Work out the finished part from the listing and answer in its coordinate system (mm). A direction names the side the tool comes from. Coordinates: 2 decimals unless noted, no trailing zeros. Loops run counter-clockwise (first coordinate to the right, second up) from the corner with the lowest first, then second, coordinate; pieces in that order, holes last. Notation, with made-up numbers: (13.5, -5.5) - (58.5, -5.5) arc R25 ccw to (58.5, 29.5) - close; hole circle Ø2 at (59.5, 47.5). An arc over 180 degrees is marked (long way). Write each question's results on one line, items separated by ' | '. Start each with the question number.
1. Find the intervals of material crossed by line 1 along Z through (x, y) = (-6, 14); line 2 along Y through (x, z) = (21, -60.5); line 3 along X through (y, z) = (-48, -6), in increasing order. Write a range as [from, to].
2. Determine the mould class of faces 6 (the cylindrical face through (-37.804, -117.535, 5.262)), 7 (the flat face through (0, 0, 0)), 8 (the cylindrical face through (-88.099, -117.535, -67.652)), 9 (the cylindrical face through (-13.186, 1.449, 1.492)) for opening direction X: released by +X, released by -X, zero draft, split by the parting line, or undercut.
3. A cutting plane is placed at B-B on z = -12.5. Determine the outline of the cut face in (x, y), then the cut area to 3 significant figures.
4. Each of these flat-tipped pins is pushed along its axis until it touches: P1, Ø3, axis at x = 10.5, y = 14, coming from the -Z side; P2, Ø10, axis at x = -28, y = -44.5, coming from the -Z side; P3, Ø5, axis at x = 7, y = -16, coming from the -Z side. Where does it stop, or does it pass through?
5. A cutting plane is placed at C-C on y = -21. Determine the outline of the cut face in (x, z).
6. A cutting plane is placed at D-D on x = 43.5. Determine the outline of the cut face in (y, z), then the cut area to 3 significant figures.
7. Which of the six approach directions +Z, -Z, +X, -X, +Y, -Y give full straight-line access (tool end or side, diameter ignored) to faces 1 (the flat face through (-93, -125, -44)), 2 (the flat face through (-0.49, -76.905, -19.72)), 3 (the cylindrical face through (6.17, -18.49, 1.49)), 4 (the flat face through (-71, -115, -46)), 5 (the flat face through (35, -59, -4))?
8. A cutting plane is placed at A-A on x = 17. Determine the outline of the cut face in (y, z).
from build123d import *

# Parameters (mm, degrees)
SKETCH1_W                     = 70
SKETCH1_H                     = 70
BOSS_EXTRUDE1_DEPTH           = 10
CBORE_FOR_M3_SHCS1_AT_2_COUNT = 2
CBORE_FOR_M3_SHCS1_AT_2_PITCH = 28.578838325
CBORE_FOR_M3_SHCS1_AT_3_COUNT = 2
CBORE_FOR_M3_SHCS1_AT_3_PITCH = 28.578838325
SKETCH14_W                    = 70
SKETCH14_H                    = 10
BOSS_EXTRUDE2_DEPTH           = 95
SKETCH13_W                    = 186
SKETCH13_H                    = 106
BOSS_EXTRUDE3_DEPTH           = 10
CHAMFER1_SIZE                 = 40
CHAMFER1_SIZE2                = 85
SKETCH18_R                    = 2.25
BOSS_EXTRUDE4_DEPTH           = 5
SKETCH19_R                    = 1.5
BOSS_EXTRUDE5_DEPTH           = 5


with BuildPart() as part:
    # Sketch1 → Boss-Extrude1 (new body)
    with BuildSketch(Plane.XY):
        Rectangle(SKETCH1_W, SKETCH1_H)
    extrude(amount=BOSS_EXTRUDE1_DEPTH)

    # Sketch4 → CBORE for M3 SHCS1 (revolve, cut)
    with BuildSketch(Plane(origin=(6.314276634, -15.244012286, 0), x_dir=(0, 1, 0), z_dir=(1, 0, 0))):
        Polygon((0, 0), (0, 10), (1.7, 10), (1.7, 3), (3.25, 3), (3.25, 0.025), (3.275, 0), align=None)
    cbore_for_m3_shcs1 = revolve(axis=Axis((6.314276634, -15.244012286, -6.35), (0, 0, 1)), mode=Mode.SUBTRACT)

    # CBORE for M3 SHCS1 at 2: CBORE for M3 SHCS1 ×2
    with Locations(*[Vector(0.13052619222005196, 0.9914448613738104, 0) * (i * CBORE_FOR_M3_SHCS1_AT_2_PITCH) for i in range(1, CBORE_FOR_M3_SHCS1_AT_2_COUNT)]):
        add(cbore_for_m3_shcs1, mode=Mode.SUBTRACT)

    # CBORE for M3 SHCS1 at 3: CBORE for M3 SHCS1 ×2
    with Locations(*[Vector(-0.7933533402912364, 0.608761429008719, 0) * (i * CBORE_FOR_M3_SHCS1_AT_3_PITCH) for i in range(1, CBORE_FOR_M3_SHCS1_AT_3_COUNT)]):
        add(cbore_for_m3_shcs1, mode=Mode.SUBTRACT)

    # Sketch14 → Boss-Extrude2 (add)
    with BuildSketch(Plane.XZ.offset(35)):
        with Locations((0, 5)):
            Rectangle(SKETCH14_W, SKETCH14_H)
    extrude(amount=BOSS_EXTRUDE2_DEPTH)

    # Sketch13 → Boss-Extrude3 (add)
    with BuildSketch(Plane.XZ.offset(130)):
        with Locations((0, -43)):
            Rectangle(SKETCH13_W, SKETCH13_H)
    extrude(amount=-BOSS_EXTRUDE3_DEPTH)

    # Chamfer1
    chamfer1_edges = [part.edges().sort_by_distance(p)[0] for p in [
        (0, -120, 0),
    ]]
    chamfer1_side = [part.faces().sort_by_distance(p)[0] for p in [
        (0, -120, -44.766933109),
    ]]
    chamfer(chamfer1_edges, length=CHAMFER1_SIZE, length2=CHAMFER1_SIZE2, reference=chamfer1_side[0])

    # Sketch18 → Boss-Extrude4 (add)
    with BuildSketch(Plane(origin=(0, -120, -115), x_dir=(1, 0, 0), z_dir=(0, 1, 0))):
        with Locations(Location((-88, -45.1, 0), (0, 0, 90))):
            Circle(SKETCH18_R)
        with Locations(Location((-44.9, -69.2, 0), (0, 0, 90))):
            Circle(SKETCH18_R)
        with Locations(Location((-72.8, -69.2, 0), (0, 0, 90))):
            Circle(SKETCH18_R)
        with Locations(Location((-88, -120, 0), (0, 0, 90))):
            Circle(SKETCH18_R)
        with Locations(Location((-39.8, -121.3, 0), (0, 0, 90))):
            Circle(SKETCH18_R)
    extrude(amount=BOSS_EXTRUDE4_DEPTH)

    # Sketch19 → Boss-Extrude5 (add)
    with BuildSketch(Plane(origin=(0, -115, 0), x_dir=(1, 0, 0), z_dir=(0, 1, 0))):
        with Locations(Location((-88, 69.9, 0), (0, 0, 270))):
            Circle(SKETCH19_R)
        with Locations(Location((-72.8, 45.8, 0), (0, 0, 270))):
            Circle(SKETCH19_R)
        with Locations(Location((-44.9, 45.8, 0), (0, 0, 270))):
            Circle(SKETCH19_R)
        with Locations(Location((-88, -5, 0), (0, 0, 270))):
            Circle(SKETCH19_R)
        with Locations(Location((-39.8, -6.3, 0), (0, 0, 270))):
            Circle(SKETCH19_R)
    extrude(amount=BOSS_EXTRUDE5_DEPTH)


solid = part.part
Values:
1) line 1: [0, 10] | line 2: [-130, -120] | line 3: [-35, 35]
2) face 6: undercut | face 7: zero draft | face 8: split by the parting line | face 9: undercut
3) outline: (-93, -130) - (93, -130) - (93, -120) - (35, -120) - (35, -61.56) - (-35, -61.56) - (-35, -120) - (-93, -120) - close | area: 5,950 mm^2
4) P1: z = 3 | P2: z = -6.82 | P3: z = 0
5) outline: (-35, 0) - (35, 0) - (35, 10) - (-35, 10) - close
6) outline: (-130, -96) - (-120, -96) - (-120, 10) - (-130, 10) - close | area: 1,060 mm^2
7) face 1: +Z, -Z, -X, +Y, -Y | face 2: -Z, +X, -X, +Y | face 3: -Z | face 4: +Y | face 5: +Z, -Z, +X, +Y
8) outline: (-130, -96) - (-120, -96) - (-120, -40) - (-35, 0) - (35, 0) - (35, 10) - (-130, 10) - close
